Autodesk Inventor part; units mm, degrees
ref_plane "Work Plane1" through (-24.9, -24.9, 7.7) normal (0, 0, 1) x (1, 0, 0)
ref_plane "YZ Plane" through (0, 0, 0) normal (1, 0, 0) x (0, 1, 0)
ref_plane "XZ Plane" through (0, 0, 0) normal (0, 1, 0) x (-1, 0, 0)
sketch "Sketch1" plane through (0, 0, 0) normal (0, 0, 1) x (1, 0, 0)
  circle A0 centre (-10, 20.9) radius 1.875
  circle A1 centre (-10, -20.9) radius 1.875
  circle A2 centre (10, 20.9) radius 1.875
  circle A3 centre (10, -20.9) radius 1.875
  circle A4 centre (20.8, -14.4) radius 2.075
  circle A5 centre (20.8, 14.4) radius 2.075
  circle A6 centre (-20.8, 14.4) radius 2.075
  circle A7 centre (-20.8, -14.4) radius 2.075
  line L0 (16.9, -16.9) -> (-16.9, -16.9)
  line L1 (-16.9, -16.9) -> (-16.9, 16.9)
  line L2 (-16.9, 16.9) -> (16.9, 16.9)
  line L3 (16.9, 16.9) -> (16.9, -16.9)
  line L4 (-17.05, 24.9) -> (-17.05, 22.55)
  line L5 (-17.05, 22.55) -> (-22.55, 17.05)
  line L6 (-22.55, 17.05) -> (-24.9, 17.05)
  line L7 (-24.9, 17.05) -> (-24.9, -17.05)
  line L8 (-24.9, -17.05) -> (-22.55, -17.05)
  line L9 (-22.55, -17.05) -> (-17.05, -22.55)
  line L10 (-17.05, -22.55) -> (-17.05, -24.9)
  line L11 (-17.05, -24.9) -> (17.05, -24.9)
  line L12 (17.05, -24.9) -> (17.05, -22.55)
  line L13 (17.05, -22.55) -> (22.55, -17.05)
  line L14 (22.55, -17.05) -> (24.9, -17.05)
  line L15 (24.9, -17.05) -> (24.9, 17.05)
  line L16 (24.9, 17.05) -> (22.55, 17.05)
  line L17 (22.55, 17.05) -> (17.05, 22.55)
  line L18 (17.05, 22.55) -> (17.05, 24.9)
  line L19 (17.05, 24.9) -> (-17.05, 24.9)
  line L20 (24.825, 16.975) -> (24.825, -16.975)
  line L21 (24.825, -16.975) -> (22.5189, -16.975)
  line L22 (22.5189, -16.975) -> (16.975, -22.5189)
  line L23 (16.975, -22.5189) -> (16.975, -24.825)
  line L24 (16.975, -24.825) -> (-16.975, -24.825)
  line L25 (-16.975, -24.825) -> (-16.975, -22.5189)
  line L26 (-16.975, -22.5189) -> (-22.5189, -16.975)
  line L27 (-22.5189, -16.975) -> (-24.825, -16.975)
  line L28 (-24.825, -16.975) -> (-24.825, 16.975)
  line L29 (-24.825, 16.975) -> (-22.5189, 16.975)
  line L30 (-22.5189, 16.975) -> (-16.975, 22.5189)
  line L31 (-16.975, 22.5189) -> (-16.975, 24.825)
  line L32 (-16.975, 24.825) -> (16.975, 24.825)
  line L33 (16.975, 24.825) -> (16.975, 22.5189)
  line L34 (16.975, 22.5189) -> (22.5189, 16.975)
  line L35 (22.5189, 16.975) -> (24.825, 16.975)
  point P0 (0, 0)
  dimension "d0" = 0.075
ref_plane "Work Plane1" through (-24.9, -24.9, 7.7) normal (0, 0, 1) x (1, 0, 0)
extrude "Extrusion1" add sketch "Sketch1" along normal blind 2.5 from surface at 7.7 contours A0 | A1 | A2 | A3 | A4 | A5 | A6 | A7 | L0 L1 L2 L3 | L20 L21 L22 L23 L24 L25 L26 L27 L28 L29 L30 L31 L32 L33 L34 L35
sketch "Sketch2" plane through (0, 0, 0) normal (0, 0, 1) x (1, 0, 0)
  line L0 (22.5189, 16.975) -> (24.825, 16.975)
  line L1 (16.975, 22.5189) -> (22.5189, 16.975)
  line L2 (16.975, 24.825) -> (16.975, 22.5189)
  line L3 (-16.975, 24.825) -> (16.975, 24.825)
  line L4 (-16.975, 22.5189) -> (-16.975, 24.825)
  line L5 (-22.5189, 16.975) -> (-16.975, 22.5189)
  line L6 (-24.825, 16.975) -> (-22.5189, 16.975)
  line L7 (-24.825, -16.975) -> (-24.825, 16.975)
  line L8 (-22.5189, -16.975) -> (-24.825, -16.975)
  line L9 (-16.975, -22.5189) -> (-22.5189, -16.975)
  line L10 (-16.975, -24.825) -> (-16.975, -22.5189)
  line L11 (16.975, -24.825) -> (-16.975, -24.825)
  line L12 (16.975, -22.5189) -> (16.975, -24.825)
  line L13 (22.5189, -16.975) -> (16.975, -22.5189)
  line L14 (24.825, -16.975) -> (22.5189, -16.975)
  line L15 (24.825, 16.975) -> (24.825, -16.975)
  line L16 (24.825, -16.975) -> (24.825, -24.825)
  line L17 (24.825, -24.825) -> (16.975, -24.825)
  line L18 (24.825, -24.825) -> (14.825, -24.825)
  line L19 (14.825, -24.825) -> (14.825, -19.825)
  line L20 (19.825, -14.825) -> (24.825, -14.825)
  line L21 (24.825, -14.825) -> (24.825, -24.825)
  line L22 (19.825, -14.825) -> (14.825, -19.825)
  line L23 (14.825, 19.825) -> (19.825, 14.825)
  line L24 (14.825, 19.825) -> (14.825, 24.825)
  line L25 (14.825, 24.825) -> (24.825, 24.825)
  line L26 (24.825, 24.825) -> (24.825, 14.825)
  line L27 (24.825, 14.825) -> (19.825, 14.825)
  line L28 (-19.825, 14.825) -> (-14.825, 19.825)
  line L29 (-19.825, 14.825) -> (-24.825, 14.825)
  line L30 (-24.825, 14.825) -> (-24.825, 24.825)
  line L31 (-24.825, 24.825) -> (-14.825, 24.825)
  line L32 (-14.825, 24.825) -> (-14.825, 19.825)
  line L33 (-14.825, -19.825) -> (-19.825, -14.825)
  line L34 (-14.825, -19.825) -> (-14.825, -24.825)
  line L35 (-14.825, -24.825) -> (-24.825, -24.825)
  line L36 (-24.825, -24.825) -> (-24.825, -14.825)
  line L37 (-24.825, -14.825) -> (-19.825, -14.825)
  line L38 (16.9, -16.9) -> (19.747, -19.747)
  line L39 (-16.9, -16.9) -> (-19.747, -19.747)
  circle A0 centre (20.8, -14.4) radius 2.075
  circle A1 centre (20.8, 14.4) radius 2.075
  circle A2 centre (-20.8, 14.4) radius 2.075
  circle A3 centre (-20.8, -14.4) radius 2.075
  line L40 (16.9, -16.9) -> (-16.9, -16.9)
  line L41 (16.9, 16.9) -> (16.9, -16.9)
  line L42 (-16.9, 16.9) -> (16.9, 16.9)
  line L43 (-16.9, -16.9) -> (-16.9, 16.9)
  line L44 (24.875, -22.9) -> (24.875, 22.9)
  arc A4 (22.9, -24.875) -> (24.875, -22.9) centre (22.9, -22.9) ccw
  line L45 (-22.9, -24.875) -> (22.9, -24.875)
  arc A5 (-24.875, -22.9) -> (-22.9, -24.875) centre (-22.9, -22.9) ccw
  line L46 (-24.875, 22.9) -> (-24.875, -22.9)
  arc A6 (-22.9, 24.875) -> (-24.875, 22.9) centre (-22.9, 22.9) ccw
  line L47 (22.9, 24.875) -> (-22.9, 24.875)
  arc A7 (24.875, 22.9) -> (22.9, 24.875) centre (22.9, 22.9) ccw
  line L48 (16.9, 16.9) -> (19.747, 19.747)
  line L49 (-16.9, 16.9) -> (-19.747, 19.747)
  line L50 (14.825, -19.825) -> (-14.825, -19.825)
  line L51 (19.825, -14.825) -> (19.825, 14.825)
  line L52 (-19.825, -14.825) -> (-19.825, 14.825)
  point P0 (0, 0)
  point P1 (14.825, -14.825)
  point P2 (17.325, -17.325)
  point P3 (-17.325, -17.325)
  point P4 (24.15, -14.825)
  point P5 (22.831, -14.825)
  point P6 (19.0838, -15.5662)
  point P7 (-19.0838, -15.5662)
  point P8 (-22.831, -14.825)
  point P9 (-24.15, -14.825)
  point P10 (-24.15, 14.825)
  point P11 (-22.831, 14.825)
  point P12 (-19.0838, 15.5662)
  point P13 (-14.825, 24.15)
  point P14 (14.825, 24.15)
  point P15 (19.0838, 15.5662)
  point P16 (22.831, 14.825)
  point P17 (24.15, 14.825)
  point P18 (-17.325, 17.325)
  point P19 (17.325, 17.325)
  point P20 (-23.3416, 24.825)
  point P21 (23.3416, 24.825)
  point P22 (-24.825, -23.3416)
  point P23 (-24.825, 23.3416)
  point P24 (23.3416, -24.825)
  point P25 (-23.3416, -24.825)
  point P26 (24.825, -23.3416)
  point P27 (24.825, 23.3416)
  dimension "d3" = 10
  dimension "d4" = 10
  dimension "d5" = 5
  dimension "d6" = 5
  dimension "d9" = 360
extrude "Extrusion2" add sketch "Sketch2" along normal blind 31.5 from surface at 10.2 contours L0 L15 L27 A1 L23 L48 L1 | L15 L20 A0 L51 A1 L27 | L15 L14 L13 L38 L22 A0 L20 | A1 L51 L27 | L27 L23 A1 | A0 L22 L20 | L20 L51 A0 | L38 L13 L12 L11 L19 L22 | L28 A2 L29 L7 L6 L5 L49 | L19 L11 L34 L50 | L39 L9 L8 L7 L37 A3 L33 | L33 L34 L11 L10 L9 L39 | L28 L29 A2 | A3 L37 L33 | L52 A2 L29 | A2 L52 A3 L37 L7 L29 | L37 A3 L52
chamfer "Chamfer1" distance 2.5 angle 45 2 edges at (17.325, 17.325, 25.95) (-17.325, 17.325, 25.95)
sketch "Sketch3" plane through (-16.975, -24.825, 7.7) normal (0, -1, 0) x (1, 0, 0)
  line L0 (-0.075, 0) -> (-0.075, 34.4)
  line L1 (34.025, 0) -> (34.025, 34.4)
  line L2 (-0.075, 17.2) -> (34.025, 17.2)
  circle A0 centre (16.975, 17.2) radius 12.75
  point P0 (16.975, -7.7)
  dimension "d16" = 25.5
extrude "Extrusion3" cut sketch "Sketch3" against normal up to surface (5 mm away)
sketch "Sketch4" plane through (-16.975, -24.825, 7.7) normal (0, -1, 0) x (1, 0, 0)
  line L0 (33.95, 34) -> (0, 34)
  line L1 (0, 0) -> (0, 34)
  line L2 (33.95, 0) -> (0, 0)
  line L3 (33.95, 0) -> (33.95, 34)
  circle A0 centre (16.975, 17.2) radius 14.5
  circle A1 centre (16.975, 17.2) radius 12.75
  point P0 (16.975, -7.7)
  dimension "d25" = 1.75
extrude "Extrusion4" add sketch "Sketch4" along normal blind 5 contours A0
chamfer "Chamfer2" distance 5 angle 45 1 edges at (-14.5, -24.825, 24.9)
properties part number "Camera Mount Side"
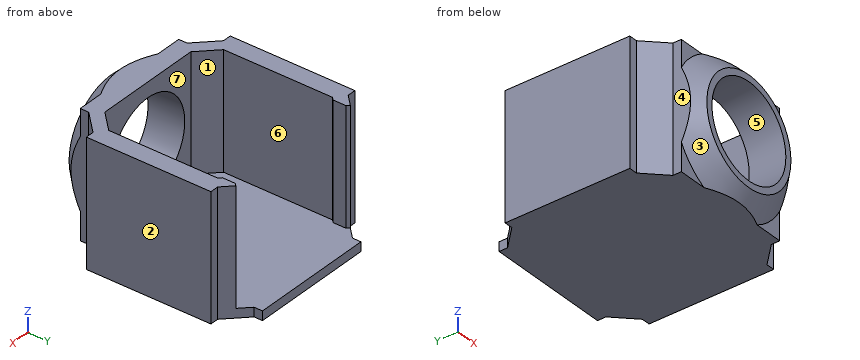
Input: part model. Units: mm. Frame: model coordinates. Face numbers are marked on the shaded views. A direction names the side the tool comes from. Give positions to 0.01 mm unless a question says otherwise; leave off trailing zeros. Loops run counter-clockwise (first coordinate to the right, second up) from the corner with the lowest first, then second, coordinate; pieces in that order, holes last. Notation, with made-up numbers: M 84.5,-18.5 L 115.5,-18.5 A12 ccw 115.5,3.5 Z; hole C 63.5,60 d10. An arc over 180 degrees is marked long. Answer as CSV lines item,"result". Start each with the question number.
1. Pin query (flat end, axial travel): P1, Ø0.7, axis at x = -23.5, z = 28.5, coming from the +Y side (3 decimals); P2, Ø0.7, axis at y = 24, z = 9.5, coming from the -X side (3 decimals); P3, Ø15, axis at x = 7, z = 27.5, coming from the +Y side (3 decimals); P4, Ø8, axis at y = -18.5, z = 13, coming from the -X side (3 decimals). Return the tip coordinate at first contact, or that it passes through.
2. Line query: L1, parallel to X at y = 3, z = 18 (3 decimals); L2, parallel to Z at x = 0, y = -27; L3, parallel to Z at x = 4, y = 4.5. Output: solid intervals per line, ascending.
3. Pull-direction query (X, two-part tool) for the marked faces 1, 2 and 3; classes: released by +X, released by -X, zero draft, split by the parting line, or undercut.
4. Section C-C on y = -18. Return loops of the section in (x, z).
5. Section A-A on x = 0. Return loops of the section in (y, z) (3 decimals), plus the area to 3 significant figures.
6. Section D-D on y = -2.5. Return loops of the section in (x, z) (3 decimals).
7. Reachability of the marked faces 4, 5, 6 and 7 from +Z, -Z, +X, -X, +Y, -Y: full face, straight path, thin tool, end or side. Return the list, or none.
Computed values:
1,P1,"stops at y = 16.975"
1,P2,"stops at x = -16.975"
1,P3,"stops at y = -19.825"
1,P4,"stops at x = -24.825"
2,L1,"x = -24.825 to -19.825, 19.825 to 24.825"
2,L2,"z = 7.7 to 12.15, 37.65 to 41.7"
2,L3,"z = 7.7 to 10.2"
3,face 1,"undercut"
3,face 2,"released by +X"
3,face 3,"split by the parting line"
4,outline,"M -21.49,7.7 L 21.49,7.7 L 21.49,41.7 L 16.65,41.7 L 16.65,10.2 L -16.65,10.2 L -16.65,41.7 L -21.49,41.7 Z"
5,outline,"M -29.825,10.4 L -27.125,7.7 L 24.825,7.7 L 24.825,10.2 L -19.825,10.2 L -19.825,12.15 L -29.825,12.15 Z; M -29.825,37.65 L -19.825,37.65 L -19.825,41.7 L -27.525,41.7 L -29.825,39.4 Z"
5,area,"190 mm²"
6,outline,"M -24.825,7.7 L 24.825,7.7 L 24.825,41.7 L 19.825,41.7 L 19.825,10.2 L -19.825,10.2 L -19.825,41.7 L -24.825,41.7 Z"
7,face 4,"+Z, -Z, -X, -Y"
7,face 5,"+Y, -Y"
7,face 6,"+Z"
7,face 7,"+Z, +Y"
